```python
from build123d import *

# Parameters (mm, degrees)
FRAME_DEPTH                = 10
SKETCH10_W                 = 145
SKETCH10_H                 = 50
CUT_EXTRUDE1_DEPTH         = 0.8
F_6_32_TAPPED_HOLE2_D      = 2.7051
F_4_40_TAPPED_HOLE1_D      = 2.2606
BOTTOM_LEGS_DEPTH          = 8.4
SIDE_ARMS_S_W              = 63
SIDE_ARMS_S_H              = 11
SIDE_ARMS_S_W_2            = 59
SIDE_ARMS_S_H_2            = 7
SIDE_ARMS_DEPTH            = 10
SIDE_TABS_S_W              = 13
SIDE_TABS_S_H              = 5.5
SIDE_TABS_S_W_2            = 9
SIDE_TABS_S_H_2            = 7
SIDE_TABS_DEPTH            = 8.4
BOTTOM_SCREWS_D            = 2.7051
LEFT_SCREW_D               = 2.7051
RIGHT_FOOT_S_W             = 7
RIGHT_FOOT_S_H             = 9.2
RIGHT_FOOT_DEPTH           = 9
RIGHT_SCREW_D              = 2.7051
CONTROL_BOARD_RELIEF_S_W   = 74.5
CONTROL_BOARD_RELIEF_S_H   = 10
CONTROL_BOARD_RELIEF_DEPTH = 2
MONITOR_SIDE_GUIDES_S_W    = 9.5
MONITOR_SIDE_GUIDES_S_H    = 11
MONITOR_SIDE_GUIDES_S_H_2  = 7
SIDE_MONITOR_GUIDES_DEPTH  = 8.4
LED_BOARD_S_W              = 35
LED_BOARD_S_H              = 10
LED_BOARD_DEPTH            = 5
F_4_CLEARANCE_HOLE1_D      = 3.2639
F_4_CLEARANCE_HOLE1_DEPTH  = 10


with BuildPart() as part:
    # Sketch1 → frame (new body)
    with BuildSketch(Plane(origin=(0, 0, 0), x_dir=(1, 0, 0), z_dir=(0, 1, 0))):
        Polygon((-72.5, 93.5), (-72.5, -93.5), (-62.5, -93.5), (-62.5, -23.5), (62.5, -23.5), (62.5, -93.5), (72.5, -93.5), (72.5, 93.5), (62.5, 93.5), (62.5, 63.5), (-62.5, 63.5), (-62.5, 93.5), align=None)
        Polygon((-62.5, -13.5), (-60.5, -13.5), (-60.5, 13.5), (-44.5, 13.5), (-44.5, -13.5), (50.5, -13.5), (50.5, 13.5), (60.5, 13.5), (60.5, -13.5), (62.5, -13.5), (62.5, 53.5), (-62.5, 53.5), align=None, mode=Mode.SUBTRACT)
    extrude(amount=FRAME_DEPTH)

    # Sketch10 → Cut-Extrude1 (cut)
    with BuildSketch(Plane(origin=(0, 10, 0), x_dir=(1, 0, 0), z_dir=(0, 1, 0))):
        with Locations((0, 68.5)):
            Rectangle(SKETCH10_W, SKETCH10_H)
    extrude(amount=-CUT_EXTRUDE1_DEPTH, mode=Mode.SUBTRACT)

    # #6-32 Tapped Hole2 (through all)
    with Locations(Plane(origin=(0, 0, 0), x_dir=(-1, 0, 0), z_dir=(0, -1, 0))):
        with Locations((55.5, -18.5), (49.8, 8.5), (-55, 8.5), (-55.5, -18.5)):
            Hole(F_6_32_TAPPED_HOLE2_D / 2)

    # #4-40 Tapped Hole1 (through all)
    with Locations(Plane(origin=(0, 0, 0), x_dir=(-1, 0, 0), z_dir=(0, -1, 0))):
        with Locations((42.25, 58.5), (-42.25, 58.5)):
            Hole(F_4_40_TAPPED_HOLE1_D / 2)

    # bottom-legs-s → bottom-legs (add)
    with BuildSketch(Plane(origin=(0, 10, 0), x_dir=(1, 0, 0), z_dir=(0, 1, 0))):
        Polygon((-72.5, -103.5), (-72.5, -82.1), (72.5, -82.1), (72.5, -103.5), (62.5, -103.5), (62.5, -93.5), (-62.5, -93.5), (-62.5, -103.5), align=None)
    extrude(amount=BOTTOM_LEGS_DEPTH)

    # side-arms-s → side-arms (add)
    with BuildSketch(Plane(origin=(0, 10, 0), x_dir=(1, 0, 0), z_dir=(0, 1, 0))):
        with Locations((-104, 28.5)):
            Rectangle(SIDE_ARMS_S_W, SIDE_ARMS_S_H)
        with Locations((102, 31)):
            Rectangle(SIDE_ARMS_S_W_2, SIDE_ARMS_S_H_2)
    extrude(amount=-SIDE_ARMS_DEPTH)

    # side-tabs-s → side-tabs (add)
    with BuildSketch(Plane(origin=(0, 10, 0), x_dir=(1, 0, 0), z_dir=(0, 1, 0))):
        with Locations((-129, 31.25)):
            Rectangle(SIDE_TABS_S_W, SIDE_TABS_S_H)
        with Locations((127, 31)):
            Rectangle(SIDE_TABS_S_W_2, SIDE_TABS_S_H_2)
    extrude(amount=SIDE_TABS_DEPTH)

    # bottom-screws (through all)
    with Locations(Plane(origin=(0, 18.4, 0), x_dir=(1, 0, 0), z_dir=(0, 1, 0))):
        with Locations((-67.5, -99.27), (67.5, -99.27)):
            Hole(BOTTOM_SCREWS_D / 2)

    # left-screw (through all)
    with Locations(Plane.XY.offset(-28.5)):
        with Locations((-129, 14.2)):
            Hole(LEFT_SCREW_D / 2)

    # right-foot-s → right-foot (add)
    with BuildSketch(Plane(origin=(131.5, 0, 0), x_dir=(0, 0, -1), z_dir=(1, 0, 0))):
        with Locations((31, 13.8)):
            Rectangle(RIGHT_FOOT_S_W, RIGHT_FOOT_S_H)
    extrude(amount=RIGHT_FOOT_DEPTH)

    # right-screw (through all)
    with Locations(Plane(origin=(0, 9.2, 0), x_dir=(-1, 0, 0), z_dir=(0, -1, 0))):
        with Locations((-135.5, 31)):
            Hole(RIGHT_SCREW_D / 2)

    # control-board-relief-s → control-board-relief (cut)
    with BuildSketch(Plane.XZ):
        with Locations((0, -58.5)):
            Rectangle(CONTROL_BOARD_RELIEF_S_W, CONTROL_BOARD_RELIEF_S_H)
    extrude(amount=-CONTROL_BOARD_RELIEF_DEPTH, mode=Mode.SUBTRACT)

    # monitor-side-guides-s → side-monitor-guides (add)
    with BuildSketch(Plane(origin=(0, 10, 0), x_dir=(1, 0, 0), z_dir=(0, 1, 0))):
        with Locations((-117.75, 28.5)):
            Rectangle(MONITOR_SIDE_GUIDES_S_W, MONITOR_SIDE_GUIDES_S_H)
        with Locations((117.75, 31)):
            Rectangle(MONITOR_SIDE_GUIDES_S_W, MONITOR_SIDE_GUIDES_S_H_2)
    extrude(amount=SIDE_MONITOR_GUIDES_DEPTH)

    # led-board-s → led-board (add)
    with BuildSketch(Plane.XZ):
        with Locations((67.5, 63.5)):
            Rectangle(LED_BOARD_S_W, LED_BOARD_S_H)
    extrude(amount=-LED_BOARD_DEPTH)

    # #4 Clearance Hole1
    with Locations(Plane(origin=(67.5, 0, 38.5), x_dir=(0, 0, -1), z_dir=(0, -1, 0))):
        with Locations((0, 0), (-25, 12.5), (-25, -12.5)):
            Hole(F_4_CLEARANCE_HOLE1_D / 2, depth=F_4_CLEARANCE_HOLE1_DEPTH)


solid = part.part
```
Geometry: final body of the model. Coordinates: model frame, mm. A direction names the side the tool comes from. Coordinates: 2 decimals unless noted, no trailing zeros. Order: outer loops, then holes, each group sorted by start corner. A loop starts at its lowest first (then second) coordinate and runs counter-clockwise, first axis right, second up. Notation, with made-up numbers: (58, 31.25) -> (109, 31.25) arc R18 ccw to (109, 49.25) -> close; hole circle Ø4 at (-18, -14.5). An arc over 180 degrees is marked (long way). Write item = value, one per line.
(1) Cut plane B-B on x = -23. Return loops of the section in (y, z), plus the area to 3 significant figures.
Solved:
outline = (0, 13.5) -> (10, 13.5) -> (10, 23.5) -> (0, 23.5) -> close; (2, -63.5) -> (9.2, -63.5) -> (9.2, -53.5) -> (2, -53.5) -> close; (10, 82.1) -> (18.4, 82.1) -> (18.4, 93.5) -> (10, 93.5) -> close
area = 268 mm²
(2) Pin query (flat end, axial travel): pin 1 Ø5.5 at (x, y) = (98, 8) entering from -Z; pin 2 Ø6.5 at (x, y) = (-128.5, 13.5) entering from +Z; pin 3 Ø2 at (y, z) = (1, -56.5) entering from +X; pin 4 Ø8 at (x, z) = (91, -41.5) entering from +Y. Return the tip coordinate at first contact, or that it passes through.
Solved:
pin_1 = -34.5
pin_2 = -28.5
pin_3 = 72.5
pin_4 = through
(3) Access query for faces 4 (the flat face through (-62.5, 5, -78)), 5 (the flat face through (-1, 2, -58)), 6 (the flat face through (-1, 10, 14)), 7 (the flat face through (113, 14, -31)), 8 (the flat face through (-122.5, 14, -26)). Directions: +Z, -Z, +X, -X, +Y, -Y. A direction counts if a zero-diameter tool reaches every point of the face in a straight line with its end or side. Return the directions, or none.
Solved:
face_4 = -Z, +Y, -Y
face_5 = -Z, -Y
face_6 = -Z, +Y
face_7 = +Z, -Z, +Y
face_8 = +Z, -X, +Y
(4) Pull-direction query (X, two-part tool) for faces 1 (the flat face through (79, 5, 62)), 2 (the flat face through (-60.5, 5, 0)), 3 (the flat face through (-135.5, 7, -30)); classes: pulls with the +X half, pulls with the -X half, needs draft (parallel to the pull), parting line crosses it, or undercut.
Solved:
face_1 = needs draft
face_2 = undercut
face_3 = pulls with the -X half
(5) Cut plane D-D on z = 30. Return loops of the section in (x, y), plus the area to 3 significant figures.
Solved:
outline = (-72.5, 0) -> (-62.5, 0) -> (-62.5, 10) -> (-72.5, 10) -> close; (62.5, 0) -> (72.5, 0) -> (72.5, 10) -> (62.5, 10) -> close
area = 200 mm²
(6) Cut plane A-A on z = -50.5. Return loops of the section in (x, y), plus the area to 3 significant figures.
Solved:
outline = (-72.5, 0) -> (-62.5, 0) -> (-62.5, 9.2) -> (-72.5, 9.2) -> close; (62.5, 0) -> (72.5, 0) -> (72.5, 9.2) -> (62.5, 9.2) -> close
area = 184 mm²
(7) Cut plane C-C on z = 3. Return loops of the section in (x, y), plus the area to 3 significant figures.
Solved:
outline = (-72.5, 0) -> (-62.5, 0) -> (-62.5, 10) -> (-72.5, 10) -> close; (-60.5, 0) -> (-44.5, 0) -> (-44.5, 10) -> (-60.5, 10) -> close; (50.5, 0) -> (60.5, 0) -> (60.5, 10) -> (50.5, 10) -> close; (62.5, 0) -> (72.5, 0) -> (72.5, 10) -> (62.5, 10) -> close
area = 460 mm²
(8) Line query: line 1 (X direction, y = 4.75, z = 38.5); line 2 (Z direction, x = 42.25, y = 4.5); line 3 (Z direction, x = 61.5, y = 1). Output: solid intervals per line, ascending.
Solved:
line_1 = -72.5 to -62.5, 62.5 to 65.87, 69.13 to 72.5
line_2 = -63.5 to -59.63, -57.37 to -53.5, 13.5 to 23.5
line_3 = -63.5 to -53.5, 13.5 to 23.5, 58.5 to 68.5
